Check sheet for the modelled part. Datum: model origin and axes. Units: mm. A direction names the side the tool comes from. Round coordinates to 2 decimals unless told otherwise and drop trailing zeros. Order: outer loops, then holes, each group sorted by start corner. A loop starts at its lowest first (then second) coordinate and runs counter-clockwise, first axis right, second up.
(1) Tool access check on faces 5 (the flat face through (-10, 4.762, -7)), 6 (the flat face through (-10, -3, 3.175)), 7 (the flat face through (0, 3, 0)), 8 (the flat face through (-20.32, -3, 7)). Record the directions out of +Z, -Z, +X, -X, +Y, -Y that give a thin tool (end or side, any length) a straight path to the whole face; none if there is none.
(2) Mould release check, pull along Z, two halves, no side actions. Record for faces 1 (the flat face through (13, 11.112, 0)), 2 (the flat face through (3, -2, -11.112)), 3 (the flat face through (-10, -3, -3.175)), 4 (the flat face through (2, -3, 11.112)): released by +Z, released by -Z, zero draft, split by the parting line, or undercut.
(3) Sectioned sample at A-A, the plane x = -2. Enter the section's corners in (y, z) (1 decimal).
(4) Thickness scan on probe 1 along Z at (x, y) = (-7, -5.25) (1 decimal); probe 2 along X at (y, z) = (8.5, 6.75); probe 3 along X at (y, z) = (0, 2.5). Record the ranges inside material, lowest first.
(5) Depth check by flat-ended pin: pin 1 (3 mm diameter, centred on x = -14.86, y = -2.22, fed in from -Z); pin 2 (1.5 mm diameter, centred on x = -5.33, y = -2.22, fed in from +Z); pin 3 (8.5 mm diameter, centred on x = -7, z = -8.5, fed in from +Y). Enter the tip coordinate at first touch or a pass-through.
(6) Sectioned sample at B-B, the plane y = 0. Enter the section's corners in (x, z) (1 decimal).
(7) Sectioned sample at C-C, the plane z = 2.25. Enter the section's corners in (x, y).
(8) Sectioned sample at D-D, the plane x = 12.7. Enter the section's corners in (y, z), and give its area (3 significant figures).
```python
from build123d import *

# Parameters (mm, degrees)
SKETCH1_W             = 22.225
SKETCH1_H             = 22.225
BOSS_EXTRUDE1_DEPTH   = 25.4
F_8_CLEARANCE_HOLE1_D = 4.4958
BOSS_EXTRUDE2_DEPTH   = 20.32
F_2_CLEARANCE_HOLE1_D = 2.4384


with BuildPart() as part:
    # Sketch1 → Boss-Extrude1 (new body)
    with BuildSketch(Plane(origin=(0, 0, 0), x_dir=(0, 0, -1), z_dir=(1, 0, 0))):
        Rectangle(SKETCH1_W, SKETCH1_H)
    extrude(amount=BOSS_EXTRUDE1_DEPTH)

    # #8 Clearance Hole1 (through all)
    with Locations(Plane(origin=(12.7, 0, 11.1125), x_dir=(0, 1, 0), z_dir=(0, 0, 1))):
        with Locations((0, 0)):
            Hole(F_8_CLEARANCE_HOLE1_D / 2)

    # Sketch3 → Boss-Extrude2 (add)
    with BuildSketch(Plane.ZY):
        Polygon((-3.175, -11.1125), (-3.175, -4.7625), (-3.175, 4.7625), (-11.1125, 4.7625), (-11.1125, -11.1125), align=None)
        Polygon((3.175, 4.7625), (3.175, -4.7625), (3.175, -11.1125), (11.1125, -11.1125), (11.1125, 4.7625), align=None)
    extrude(amount=BOSS_EXTRUDE2_DEPTH)

    # #2 Clearance Hole1 (through all)
    with Locations(Plane(origin=(0, 0, -11.1125), x_dir=(-1, 0, 0), z_dir=(0, 0, -1))):
        with Locations((5.334, -2.2225), (14.859, -2.2225)):
            Hole(F_2_CLEARANCE_HOLE1_D / 2)


solid = part.part
```
Derived:
1. face 5: +Z, -Z, -X, +Y
1. face 6: -X, +Y, -Y
1. face 7: -X, +Y
1. face 8: +Z, -Z, -X, +Y, -Y
2. face 1: zero draft
2. face 2: released by -Z
2. face 3: undercut
2. face 4: released by +Z
3. outline: (-11.1, -11.1) - (4.8, -11.1) - (4.8, -3.2) - (-11.1, -3.2) - close; (-11.1, 3.2) - (4.8, 3.2) - (4.8, 11.1) - (-11.1, 11.1) - close
4. probe 1: z = -11.1 to -3.2, 3.2 to 11.1
4. probe 2: x = 0 to 25.4
4. probe 3: x = 0 to 10.45, 14.95 to 25.4
5. pin 1: stops at z = -11.11
5. pin 2: passes through
5. pin 3: stops at y = 4.76
6. outline: (-20.3, -11.1) - (10.5, -11.1) - (10.5, 11.1) - (-20.3, 11.1) - (-20.3, 3.2) - (0, 3.2) - (0, -3.2) - (-20.3, -3.2) - close; (14.9, -11.1) - (25.4, -11.1) - (25.4, 11.1) - (14.9, 11.1) - close
7. outline: (0, -11.11) - (25.4, -11.11) - (25.4, 11.11) - (0, 11.11) - close; hole circle Ø4.5 at (12.7, 0)
8. outline: (-11.11, -11.11) - (-2.25, -11.11) - (-2.25, 11.11) - (-11.11, 11.11) - close; (2.25, -11.11) - (11.11, -11.11) - (11.11, 11.11) - (2.25, 11.11) - close
8. area: 394 mm2
